Source: CAD feature listing. Evaluate the final solid. Frame: model axes, mm. A direction names the side the tool comes from. Coordinates: 2 decimals unless noted, no trailing zeros. Loops run counter-clockwise (first coordinate to the right, second up) from the corner with the lowest first, then second, coordinate; pieces in that order, holes last.
```python
from build123d import *

# Parameters (mm, degrees)
SKETCH1_W           = 300
SKETCH1_H           = 300
BOSS_EXTRUDE1_DEPTH = 30
SKETCH2_W           = 210
SKETCH2_H           = 210
CUT_EXTRUDE1_DEPTH  = 25
SKETCH6_R           = 25
BOSS_EXTRUDE3_DEPTH = 24
SKETCH4_R           = 1.5
CUT_EXTRUDE3_DEPTH  = 5
CUT_EXTRUDE4_DEPTH  = 15
FILLET1_R           = 105
SKETCH5_R           = 125
SKETCH5_R_2         = 112.5
BOSS_EXTRUDE2_DEPTH = 30
FILLET5_R           = 7.5
FILLET6_R           = 5
FILLET7_R           = 100


with BuildPart() as part:
    # Sketch1 → Boss-Extrude1 (new body)
    with BuildSketch(Plane(origin=(0, 0, 0), x_dir=(1, 0, 0), z_dir=(0, 1, 0))):
        Rectangle(SKETCH1_W, SKETCH1_H)
    extrude(amount=BOSS_EXTRUDE1_DEPTH)

    # Sketch2 → Cut-Extrude1 (cut)
    with BuildSketch(Plane(origin=(0, 30, 0), x_dir=(1, 0, 0), z_dir=(0, 1, 0))):
        Rectangle(SKETCH2_W, SKETCH2_H)
    extrude(amount=-CUT_EXTRUDE1_DEPTH, mode=Mode.SUBTRACT)

    # Sketch6 → Boss-Extrude3 (add)
    with BuildSketch(Plane(origin=(0, 5, 0), x_dir=(1, 0, 0), z_dir=(0, 1, 0))):
        with Locations(Location((0, 0, 0), (0, 0, 270))):
            Circle(SKETCH6_R)
    extrude(amount=BOSS_EXTRUDE3_DEPTH)

    # Sketch4 → Cut-Extrude3 (cut)
    with BuildSketch(Plane(origin=(0, 5, 0), x_dir=(1, 0, 0), z_dir=(0, 1, 0))):
        with Locations(Location((90, 10, 0), (0, 0, 270))):
            Circle(SKETCH4_R)
        with Locations(Location((90, -10, 0), (0, 0, 90))):
            Circle(SKETCH4_R)
        with Locations(Location((70, -10, 0), (0, 0, 270))):
            Circle(SKETCH4_R)
        with Locations(Location((70, 10, 0), (0, 0, 90))):
            Circle(SKETCH4_R)
        with Locations(Location((-90, -10, 0), (0, 0, 270))):
            Circle(SKETCH4_R)
        with Locations(Location((-70, -10, 0), (0, 0, 90))):
            Circle(SKETCH4_R)
        with Locations(Location((-70, 10, 0), (0, 0, 270))):
            Circle(SKETCH4_R)
        with Locations(Location((-90, 10, 0), (0, 0, 90))):
            Circle(SKETCH4_R)
        with Locations(Location((10, -70, 0), (0, 0, 90))):
            Circle(SKETCH4_R)
        with Locations(Location((10, -90, 0), (0, 0, 270))):
            Circle(SKETCH4_R)
        with Locations(Location((-10, -90, 0), (0, 0, 90))):
            Circle(SKETCH4_R)
        with Locations(Location((-10, -70, 0), (0, 0, 270))):
            Circle(SKETCH4_R)
        with Locations(Location((10, 70, 0), (0, 0, 270))):
            Circle(SKETCH4_R)
        with Locations(Location((10, 90, 0), (0, 0, 90))):
            Circle(SKETCH4_R)
        with Locations(Location((-10, 70, 0), (0, 0, 90))):
            Circle(SKETCH4_R)
        with Locations(Location((-10, 90, 0), (0, 0, 270))):
            Circle(SKETCH4_R)
    extrude(amount=-CUT_EXTRUDE3_DEPTH, mode=Mode.SUBTRACT)

    # Sketch7 → Cut-Extrude4 (cut)
    with BuildSketch(Plane(origin=(0, 29, 0), x_dir=(1, 0, 0), z_dir=(0, 1, 0))):
        with BuildLine():
            Line((-2.100270755, -1.356046738), (0.899729245, -2.332485217))
            ThreePointArc((0.899729245, -2.332485217), (2.061470726, -1.414333215), (2.5, 0))
            ThreePointArc((2.5, 0), (-0.706867425, 2.397986331), (-2.100270755, -1.356046738))
        make_face()
    extrude(amount=-CUT_EXTRUDE4_DEPTH, mode=Mode.SUBTRACT)

    # Fillet1
    fillet1_edges = [part.edges().sort_by_distance(p)[0] for p in [
        (-105, 17.5, 105),
        (105, 17.5, 105),
        (105, 17.5, -105),
        (-105, 17.5, -105),
    ]]
    fillet(fillet1_edges, radius=FILLET1_R - 0.0001)  # a hair under: the kernel refuses the full size

    # Sketch5 → Boss-Extrude2 (add)
    with BuildSketch(Plane(origin=(0, 30, 0), x_dir=(1, 0, 0), z_dir=(0, 1, 0))):
        with Locations(Location((0, 0, 0), (0, 0, 90))):
            Circle(SKETCH5_R)
        with Locations(Location((0, 0, 0), (0, 0, 270))):
            Circle(SKETCH5_R_2, mode=Mode.SUBTRACT)
    extrude(amount=BOSS_EXTRUDE2_DEPTH)

    # Fillet5
    fillet5_edges = [part.edges().sort_by_distance(p)[0] for p in [
        (0, 30, -112.5),
    ]]
    fillet(fillet5_edges, radius=FILLET5_R - 0.0001)  # a hair under: the kernel refuses the full size

    # Fillet6
    fillet6_edges = [part.edges().sort_by_distance(p)[0] for p in [
        (0, 60, 125),
        (0, 60, -112.5),
    ]]
    fillet(fillet6_edges, radius=FILLET6_R)

    # Chamfer1: read off the stored shape, not the designer's step
    # Chamfer1 outline → Chamfer1 (revolve)
    with BuildSketch(Plane.XY):
        Polygon((124.670923067, 56.783950028), (124.670923067, 55), (125, 55), (125, 30), (148.025538402, 30), align=None)
    revolve(axis=Axis((0, 0, 0), (0, 1, 0)))

    # Fillet7
    fillet7_edges = [part.edges().sort_by_distance(p)[0] for p in [
        (150, 15, 150),
        (-150, 15, 150),
        (-150, 15, -150),
        (150, 15, -150),
    ]]
    fillet(fillet7_edges, radius=FILLET7_R)


solid = part.part
```
Q1. First-contact query: pin 1 Ø3 at (x, z) = (86.5, -75) entering from +Y; pin 2 Ø15 at (x, z) = (12, -5.5) entering from +Y; pin 3 Ø4 at (x, z) = (10, 70) entering from +Y. Flat tips, straight axial feed; report the tip coordinate or a pass-through.
Q2. Section query A-A on y = 43. Return the cut outline in (x, z).
Q3. Draft query along X for faces 3 (the cylindrical face through (4.95, 46.13, -112.39)), 4 (the flat face through (79, 60, -88)), 5 (the conical face through (-27.272, 55.483, 122.813)). Return one class per face: released by +X, released by -X, zero draft, split by the parting line, or undercut.
Q4. Material intervals for line 1 along X through (y, z) = (2.55, 70); line 2 along X through (y, z) = (2.4, 90), sorted ascending.
Q5. Reachability of faces 1 (the flat face through (-2, 0, -2)), 2 (the cylindrical face through (75.058, 17.325, -73.425)) from +Z, -Z, +X, -X, +Y, -Y: full face, straight path, thin tool, end or side. Return the list, or none.
Resolved:
1. pin 1: stops at y = 59.77
1. pin 2: stops at y = 29
1. pin 3: stops at y = 5
2. outline: circle Ø273.38 at (0, 0); hole circle Ø225 at (0, 0)
3. face 3: undercut
3. face 4: zero draft
3. face 5: split by the parting line
4. line 1: x = -147.98 to -11.5, -8.5 to 8.5, 11.5 to 147.98
4. line 2: x = -141.65 to -11.5, -8.5 to 8.5, 11.5 to 141.65
5. face 1: +Z, -Z, +X, -X, -Y
5. face 2: +Y
